Design review of the part built by this model. Coordinates are the model's own, in mm. A direction names the side the tool comes from. Give positions to 0.01 mm unless a question says otherwise; leave off trailing zeros. Write each loop counter-clockwise with the first axis right and the second up, starting at its lowest first coordinate (ties: lowest second). Pieces come first, ordered by that corner, then holes. Notation, with made-up numbers: (89, 57.25) -> (113, 57.25) arc R13 ccw to (113, 61.25) -> close; hole circle Ø11 at (24, 44.5). An arc over 180 degrees is marked (long way). Write each question's results on one line, items separated by ' | '. Start each with the question number.
(1) For faces 5 (the face through (-21, -11.5, -4)), 6 (the face through (0, 0, 0)), 7 (the face through (-0.392, 10.359, 1.797)), 8 (the face through (-31, -13, -1)), list the 3-axis set-ups (+Z, -Z, +X, -X, +Y, -Y) from which the entire face can be reached by the end or side of a thin tool; tool diameter is ignored.
(2) Take a section at A-A (x = 12). State the section outline as (y, z) points.
(3) Mouldability with a two-part tool opening along Y and no side actions: class faces 1 (the face through (31.5, -0.1, 6.9)), 2 (the face through (0, -5, 3)), 3 (the face through (-32.33, -12.25, -17.33)), 4 (the face through (-33.028, -8.655, -13.921)) as released by +Y, released by -Y, zero draft, split by the parting line, or undercut.
(4) Take a section at B-B (z = -16.5). State the section outline as (x, y) points, plus the area to 3 significant figures.
(5) Clearance check with flat-ended pins moving along their axes: pin 1 (3 mm diameter, centred on x = 9, y = 4.5, fed in from +Z); pin 2 (5 mm diameter, centred on x = 27, y = 1, fed in from -Z); pin 3 (6.5 mm diameter, centred on x = -25.5, z = 5.5, fed in from -Y). State where each tip first meets the part, or that it passes through.
(6) To check wall thickness, follow probe 1 along X at (y, z) = (2, -17); probe 2 along Y at (x, z) = (-31.5, 9.25); probe 3 along X at (y, z) = (-11, 9). State the ranges of each line that lie inside material, in increasing order.
(7) Take a section at C-C (z = -10). State the section outline as (x, y) points, plus the area to 3 significant figures.
from build123d import *

# Parameters (mm, degrees)
SKETCH1_W                                  = 70
SKETCH1_H                                  = 15
BOSS_EXTRUDE1_DEPTH                        = 3
SKETCH2_W                                  = 7
SKETCH2_H                                  = 15
BOSS_EXTRUDE2_DEPTH                        = 10
SKETCH5_R                                  = 4.5
CUT_EXTRUDE1_DEPTH                         = 72.590851371
SKETCH6_R                                  = 6.1
CUT_EXTRUDE4_DEPTH                         = 2.1
BOSS_EXTRUDE3_DEPTH                        = 13
SKETCH8_R                                  = 2
CUT_EXTRUDE5_DEPTH                         = 40.534794802
SKETCH9_R                                  = 1.75
CUT_EXTRUDE6_DEPTH                         = 39.65229618
MIRROR1_AT_THE_SECOND_PLANE_COPY_1_SKETC_R = 6.1
MIRROR1_AT_THE_SECOND_PLANE_COPY_1_DEPTH   = 2.1
MIRROR1_AT_THE_SECOND_PLANE_COPY_2_DEPTH   = 13
MIRROR1_AT_THE_SECOND_PLANE_COPY_3_SKETC_R = 2
MIRROR1_AT_THE_SECOND_PLANE_COPY_3_DEPTH   = 40.534794802
MIRROR1_AT_THE_SECOND_PLANE_COPY_4_SKETC_R = 1.75
MIRROR1_AT_THE_SECOND_PLANE_COPY_4_DEPTH   = 39.65229618
FILLET1_R                                  = 6
SKETCH10_W                                 = 56
SKETCH10_H                                 = 23
BOSS_EXTRUDE4_DEPTH                        = 15
FILLET2_R                                  = 4
SKETCH11_R                                 = 13
CUT_EXTRUDE7_DEPTH                         = 66.627738058
SKETCH14_W                                 = 7
SKETCH14_H                                 = 26
BOSS_EXTRUDE6_DEPTH                        = 5
SKETCH15_W                                 = 7
SKETCH15_H                                 = 26
BOSS_EXTRUDE7_DEPTH                        = 14
FILLET5_R                                  = 4
SKETCH16_R                                 = 5.5
CUT_EXTRUDE9_DEPTH                         = 74.688533708
FILLET5_OF_MIRROR2_R                       = 4
SKETCH17_R                                 = 1.25
CUT_EXTRUDE10_DEPTH                        = 74.688533708
CUT_EXTRUDE14_DEPTH                        = 31
CUT_EXTRUDE14_DEPTH_BACK                   = 31
SKETCH18_R                                 = 12.95
SKETCH19_W                                 = 30
SKETCH19_H                                 = 10
BOSS_EXTRUDE8_DEPTH                        = 5
BOSS_EXTRUDE8_DIRECTION_2_REACH            = 48.757
SKETCH20_R                                 = 2
CUT_EXTRUDE15_DEPTH                        = 10
SKETCH21_R                                 = 1.75
CUT_EXTRUDE16_DEPTH                        = 45.511234574


with BuildPart() as part:
    # Sketch1 → Boss-Extrude1 (new body)
    with BuildSketch(Plane.XY):
        Rectangle(SKETCH1_W, SKETCH1_H)
    extrude(amount=BOSS_EXTRUDE1_DEPTH)

    # Sketch2 → Boss-Extrude2 (add)
    with BuildSketch(Plane.XY.offset(3)):
        with Locations((-31.5, 0)):
            Rectangle(SKETCH2_W, SKETCH2_H)
        with Locations((31.5, 0)):
            Rectangle(SKETCH2_W, SKETCH2_H)
    extrude(amount=BOSS_EXTRUDE2_DEPTH)

    # Sketch5 → Cut-Extrude1 (cut, through all)
    with BuildSketch(Plane(origin=(35, 0, 0), x_dir=(0, 0, -1), z_dir=(1, 0, 0))):
        with Locations((-13, 0)):
            Circle(SKETCH5_R)
    extrude(amount=-CUT_EXTRUDE1_DEPTH, mode=Mode.SUBTRACT)

    # Sketch6 → Cut-Extrude4 (cut, symmetric)
    with BuildSketch(Plane(origin=(31.5, 0, 0), x_dir=(0, 0, -1), z_dir=(1, 0, 0))):
        with Locations((-13, 0)):
            Circle(SKETCH6_R)
    cut_extrude4 = extrude(amount=CUT_EXTRUDE4_DEPTH, both=True, mode=Mode.SUBTRACT)

    # Sketch7 → Boss-Extrude3 (add)
    with BuildSketch(Plane.XY):
        Polygon((28, 8.1), (28, 13), (35, 13), (35, 8.1), (35, 4.5), (33.6, 4.5), (33.6, 6.1), (29.4, 6.1), (29.4, 4.5), (28, 4.5), align=None)
    boss_extrude3 = extrude(amount=BOSS_EXTRUDE3_DEPTH)

    # Sketch8 → Cut-Extrude5 (cut, symmetric)
    with BuildSketch(Plane.XY.offset(13)):
        with Locations((31.5, 10)):
            Circle(SKETCH8_R)
    cut_extrude5 = extrude(amount=CUT_EXTRUDE5_DEPTH, both=True, mode=Mode.SUBTRACT)

    # Sketch9 → Cut-Extrude6 (cut, through all)
    with BuildSketch(Plane.XY.offset(3)):
        with Locations((-10, -4)):
            Circle(SKETCH9_R)
    cut_extrude6 = extrude(amount=-CUT_EXTRUDE6_DEPTH, mode=Mode.SUBTRACT)

    # Mirror1: Cut-Extrude4, Boss-Extrude3, Cut-Extrude5, Cut-Extrude6 across plane
    add(cut_extrude4.mirror(Plane(origin=(0, 0, 0), x_dir=(0, 0, 1), z_dir=(1, 0, 0))), mode=Mode.SUBTRACT)
    add(boss_extrude3.mirror(Plane(origin=(0, 0, 0), x_dir=(0, 0, 1), z_dir=(1, 0, 0))))
    add(cut_extrude5.mirror(Plane(origin=(0, 0, 0), x_dir=(0, 0, 1), z_dir=(1, 0, 0))), mode=Mode.SUBTRACT)
    add(cut_extrude6.mirror(Plane(origin=(0, 0, 0), x_dir=(0, 0, 1), z_dir=(1, 0, 0))), mode=Mode.SUBTRACT)

    # Mirror1 at the second plane: Cut-Extrude4, Boss-Extrude3, Cut-Extrude5, Cut-Extrude6 across plane
    add(cut_extrude4.mirror(Plane.ZX), mode=Mode.SUBTRACT)
    add(boss_extrude3.mirror(Plane.ZX))
    add(cut_extrude5.mirror(Plane.ZX), mode=Mode.SUBTRACT)
    add(cut_extrude6.mirror(Plane.ZX), mode=Mode.SUBTRACT)

    # Mirror1 at the second plane copy 1 sketc → Mirror1 at the second plane copy 1 (cut, symmetric)
    with BuildSketch(Plane(origin=(-31.5, 0, 0), x_dir=(0, 0, -1), z_dir=(-1, 0, 0))):
        with Locations((-13, 0)):
            Circle(MIRROR1_AT_THE_SECOND_PLANE_COPY_1_SKETC_R)
    extrude(amount=MIRROR1_AT_THE_SECOND_PLANE_COPY_1_DEPTH, both=True, mode=Mode.SUBTRACT)

    # Mirror1 at the second plane copy 2 sketc → Mirror1 at the second plane copy 2 (add)
    with BuildSketch(Plane(origin=(0, 0, 0), x_dir=(-1, 0, 0), z_dir=(0, 0, 1))):
        Polygon((28, 8.1), (28, 13), (35, 13), (35, 8.1), (35, 4.5), (33.6, 4.5), (33.6, 6.1), (29.4, 6.1), (29.4, 4.5), (28, 4.5), align=None)
    extrude(amount=MIRROR1_AT_THE_SECOND_PLANE_COPY_2_DEPTH)

    # Mirror1 at the second plane copy 3 sketc → Mirror1 at the second plane copy 3 (cut, symmetric)
    with BuildSketch(Plane(origin=(0, 0, 13), x_dir=(-1, 0, 0), z_dir=(0, 0, 1))):
        with Locations((31.5, 10)):
            Circle(MIRROR1_AT_THE_SECOND_PLANE_COPY_3_SKETC_R)
    extrude(amount=MIRROR1_AT_THE_SECOND_PLANE_COPY_3_DEPTH, both=True, mode=Mode.SUBTRACT)

    # Mirror1 at the second plane copy 4 sketc → Mirror1 at the second plane copy 4 (cut, through all)
    with BuildSketch(Plane(origin=(0, 0, 3), x_dir=(-1, 0, 0), z_dir=(0, 0, 1))):
        with Locations((-10, -4)):
            Circle(MIRROR1_AT_THE_SECOND_PLANE_COPY_4_SKETC_R)
    extrude(amount=-MIRROR1_AT_THE_SECOND_PLANE_COPY_4_DEPTH, mode=Mode.SUBTRACT)

    # Fillet1
    fillet1_edges = [part.edges().sort_by_distance(p)[0] for p in [
        (-28, 0, 3),
        (28, 0, 3),
    ]]
    fillet(fillet1_edges, radius=FILLET1_R)

    # Sketch10 → Boss-Extrude4 (add)
    with BuildSketch(Plane(origin=(0, 0, 3), x_dir=(-1, 0, 0), z_dir=(0, 0, -1))):
        Rectangle(SKETCH10_W, SKETCH10_H)
    extrude(amount=BOSS_EXTRUDE4_DEPTH)

    # Fillet2
    # the kernel refuses this fillet: 4 mm, written as the material it takes off along each edge
    with BuildSketch(Plane(origin=(-28, 11.5, 3), x_dir=(0, 0, -1), z_dir=(1, 0, 0)), Plane(origin=(28, -11.5, 3), x_dir=(0, 0, -1), z_dir=(-1, 0, 0))) as fillet2_piece_1:
        with BuildLine():
            CenterArc((FILLET2_R, -FILLET2_R), FILLET2_R, 90, 90)
            Line((0, -FILLET2_R), (0, 0))
            Line((0, 0), (FILLET2_R, 0))
        make_face()
    extrude(amount=56, mode=Mode.SUBTRACT)

    # Sketch11 → Cut-Extrude7 (cut, through all)
    with BuildSketch(Plane(origin=(28, 0, 0), x_dir=(0, 0, -1), z_dir=(1, 0, 0))):
        with Locations((13, 0)):
            Circle(SKETCH11_R)
    extrude(amount=-CUT_EXTRUDE7_DEPTH, mode=Mode.SUBTRACT)

    # Sketch14 → Boss-Extrude6 (add)
    with BuildSketch(Plane(origin=(0, 0, 0), x_dir=(-1, 0, 0), z_dir=(0, 0, -1))):
        with Locations((31.5, 0)):
            Rectangle(SKETCH14_W, SKETCH14_H)
    boss_extrude6 = extrude(amount=BOSS_EXTRUDE6_DEPTH)

    # Sketch15 → Boss-Extrude7 (add)
    with BuildSketch(Plane(origin=(0, 0, -5), x_dir=(-1, 0, 0), z_dir=(0, 0, -1))):
        with Locations((31.5, 0)):
            Rectangle(SKETCH15_W, SKETCH15_H)
    boss_extrude7 = extrude(amount=BOSS_EXTRUDE7_DEPTH)

    # Fillet5
    fillet5_edges = [part.edges().sort_by_distance(p)[0] for p in [
        (-31.5, 13, -19),
        (-31.5, -13, -19),
    ]]
    fillet(fillet5_edges, radius=FILLET5_R)

    # Sketch16 → Cut-Extrude9 (cut, through all)
    with BuildSketch(Plane.ZY.offset(35)):
        with Locations((-10, 0)):
            Circle(SKETCH16_R)
    cut_extrude9 = extrude(amount=-CUT_EXTRUDE9_DEPTH, mode=Mode.SUBTRACT)

    # Mirror2: Boss-Extrude6, Boss-Extrude7, Cut-Extrude9 across plane
    add(boss_extrude6.mirror(Plane(origin=(0, 0, 0), x_dir=(0, 0, 1), z_dir=(1, 0, 0))))
    add(boss_extrude7.mirror(Plane(origin=(0, 0, 0), x_dir=(0, 0, 1), z_dir=(1, 0, 0))))
    add(cut_extrude9.mirror(Plane(origin=(0, 0, 0), x_dir=(0, 0, 1), z_dir=(1, 0, 0))), mode=Mode.SUBTRACT)

    # Fillet5 of Mirror2
    fillet5_of_mirror2_edges = [part.edges().sort_by_distance(p)[0] for p in [
        (31.5, 13, -19),
        (31.5, -13, -19),
    ]]
    fillet(fillet5_of_mirror2_edges, radius=FILLET5_OF_MIRROR2_R)

    # Sketch17 → Cut-Extrude10 (cut, through all)
    with BuildSketch(Plane.ZY.offset(35)):
        with Locations((-13, 9.5)):
            Circle(SKETCH17_R)
        with Locations((-13, -9.5)):
            Circle(SKETCH17_R)
    extrude(amount=-CUT_EXTRUDE10_DEPTH, mode=Mode.SUBTRACT)

    # Sketch18 → Cut-Extrude14 (cut, two sides: drawn at the far end of the back side and taken through both)
    with BuildSketch(Plane(origin=(0, 0, 0), x_dir=(0, 0, -1), z_dir=(1, 0, 0)).offset(-CUT_EXTRUDE14_DEPTH_BACK)):
        with Locations((13, 0)):
            Circle(SKETCH18_R)
    extrude(amount=CUT_EXTRUDE14_DEPTH + CUT_EXTRUDE14_DEPTH_BACK, mode=Mode.SUBTRACT)

    # Sketch19 → Boss-Extrude8 (add)
    with BuildSketch(Plane.XZ.offset(11.5)):
        with Locations((0, -2)):
            Rectangle(SKETCH19_W, SKETCH19_H)
    extrude(amount=BOSS_EXTRUDE8_DEPTH)

    # Sketch19 → Boss-Extrude8 direction 2 (add, up to next)
    with BuildSketch(Plane.XZ.offset(11.5), mode=Mode.PRIVATE) as boss_extrude8_direction_2_sk1:
        with Locations((0, -2)):
            Rectangle(SKETCH19_W, SKETCH19_H)
    boss_extrude8_direction_2_tool1 = extrude(boss_extrude8_direction_2_sk1.sketch, amount=-BOSS_EXTRUDE8_DIRECTION_2_REACH, mode=Mode.PRIVATE) - part.part
    add(boss_extrude8_direction_2_tool1.solids().sort_by_distance((0, -11.5, -2))[0])

    # Sketch20 → Cut-Extrude15 (cut)
    with BuildSketch(Plane.XZ.offset(16.5)):
        with Locations(Location((-8.5, -3, 0), (0, 0, 270))):
            Circle(SKETCH20_R)
        with Locations(Location((8.5, -3, 0), (0, 0, 270))):
            Circle(SKETCH20_R)
    extrude(amount=-CUT_EXTRUDE15_DEPTH, mode=Mode.SUBTRACT)

    # Sketch21 → Cut-Extrude16 (cut, through all)
    with BuildSketch(Plane.XY.offset(3)):
        with Locations((0, -11.5)):
            Circle(SKETCH21_R)
    extrude(amount=-CUT_EXTRUDE16_DEPTH, mode=Mode.SUBTRACT)


solid = part.part
Report:
1) face 5: +Z, -Z, -Y | face 6: -Z | face 7: +Z, +Y | face 8: +Z, -Z, -X, -Y
2) outline: (-16.5, -7) -> (-11.5, -7) -> (-11.5, -6.94) arc R13 cw to (11.5, -6.94) -> (11.5, -1) arc R4 ccw to (7.5, 3) -> (-16.5, 3) -> close
3) face 1: undercut | face 2: zero draft | face 3: released by -Y | face 4: undercut
4) outline: (-35, -12.71) -> (-28, -12.71) -> (-28, -12.47) -> (-31, -12.47) -> (-31, 12.47) -> (-28, 12.47) -> (-28, 12.71) -> (-35, 12.71) -> close; (28, -12.71) -> (35, -12.71) -> (35, 12.71) -> (28, 12.71) -> (28, 12.47) -> (31, 12.47) -> (31, -12.47) -> (28, -12.47) -> close | area: 206 mm2
5) pin 1: z = 3 | pin 2: z = -0.48 | pin 3: y = -13
6) probe 1: -35 to -31, 31 to 35 | probe 2: -13 to -12, -8 to -4.81, 4.81 to 8, 12 to 13 | probe 3: -35 to -33.23, -29.77 to -28, 28 to 29.77, 33.23 to 35
7) outline: (-35, -13) -> (-28, -13) -> (-28, -12.6) -> (-31, -12.6) -> (-31, -5.5) -> (-35, -5.5) -> close; (-35, 5.5) -> (-31, 5.5) -> (-31, 12.6) -> (-28, 12.6) -> (-28, 13) -> (-35, 13) -> close; (28, -13) -> (35, -13) -> (35, -5.5) -> (31, -5.5) -> (31, -12.6) -> (28, -12.6) -> close; (28, 12.6) -> (31, 12.6) -> (31, 5.5) -> (35, 5.5) -> (35, 13) -> (28, 13) -> close | area: 125 mm2
